Source: three-view drawing plus pictorial views. Frame: mm from the lowest corner of the part. A direction names the side the tool comes from. Give positions to 0.01 mm unless a question says otherwise; leave off trailing zeros. Loops run counter-clockwise (first coordinate to the right, second up) from the corner with the lowest first, then second, coordinate; pieces in that order, holes last. Notation, with made-up numbers: (24, 62.25) -> (46, 62.25) arc R6 cw to (46, 69.25) -> close; hole circle Ø8 at (34.5, 58). An arc over 180 degrees is marked (long way). One line per item, written item: value. Start each with the question number.
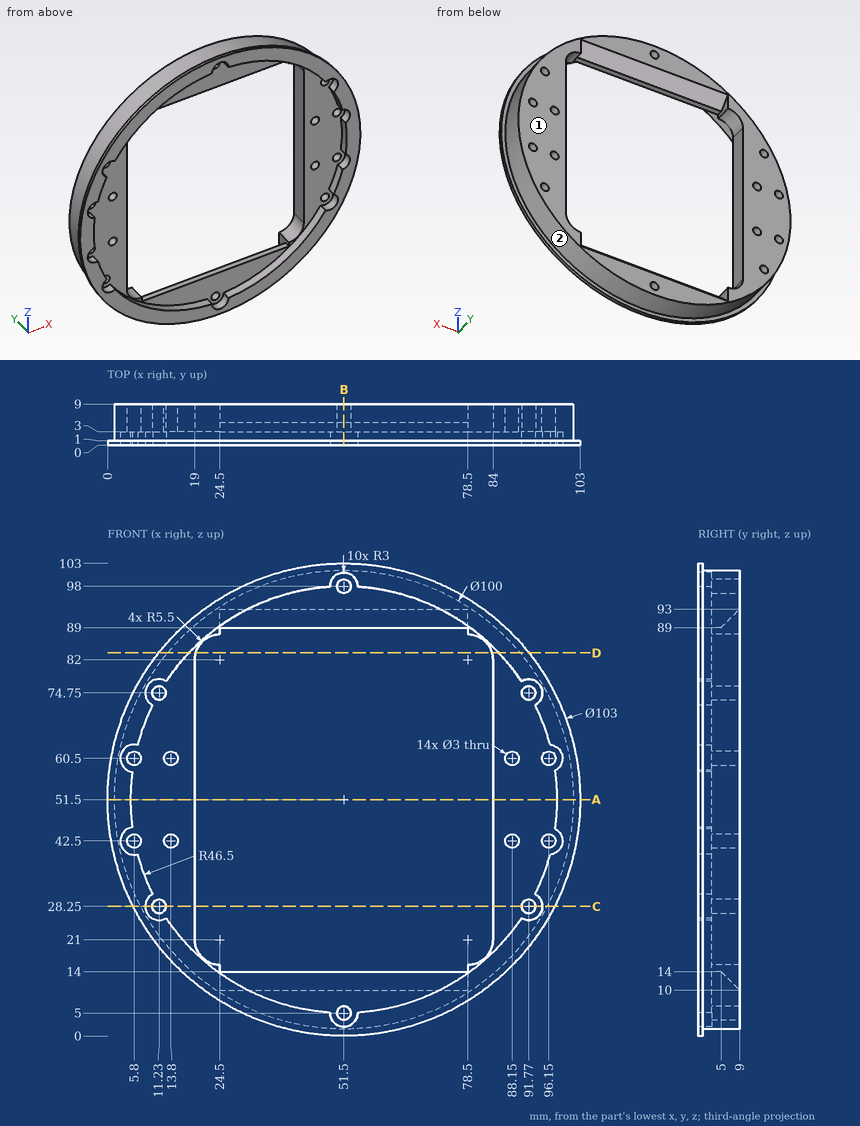
Item 1: Section A-A, the plane z = 51.5. Output: boundary loops of the cut face in (x, y).
Item 2: Section D-D, the plane z = 83.5. Output: boundary loops of the cut face in (x, y), then the cut area to 4 significant figures.
Item 3: Section C-C, the plane z = 28.25. Output: boundary loops of the cut face in (x, y).
Item 4: Pin query (flat end, axial travel): pin 1 (4 mm diameter, centred on x = 51.5, z = 5, fed in from -Y); pin 2 (1.6 mm diameter, centred on x = 44, y = 4, fed in from -Z); pin 3 (4.5 mm diameter, centred on y = 7, z = 13, fed in from -X); pin 4 (12 mm diameter, centred on x = 36.5, z = 81, fed in from -Y). Return the tip coordinate at first contact, or that it passes through.
Item 5: Ray query, line 1 along Z through (x, y) = (96.15, 7.65); line 2 along X through (y, z) = (4.5, 37.5); line 3 along Z through (x, y) = (5.8, 6.8) (1 decimal). Return the intervals inside material, ascending. Write a range as [from, to].
Item 6: Access query for the marked faces 1 and 2. Directions: +Z, -Z, +X, -X, +Y, -Y. A direction counts if a zero-diameter tool reaches every point of the face in a straight line with its end or side. Return the directions, or none.
Item 7: Section B-B, the plane x = 51.5. Output: boundary loops of the cut face in (y, z), then the cut area to 3 significant figures.
Geometry check:
1. outline: (0, 0) -> (5, 0) -> (5, 3) -> (19, 3) -> (19, 9) -> (1.5, 9) -> (1.5, 1) -> (0, 1) -> close; (84, 3) -> (98, 3) -> (98, 0) -> (103, 0) -> (103, 1) -> (101.5, 1) -> (101.5, 9) -> (84, 9) -> close
2. outline: (11.15, 0) -> (17.76, 0) -> (17.76, 3) -> (19.21, 3) -> (19.21, 9) -> (13.08, 9) -> (13.08, 1) -> (11.15, 1) -> close; (83.79, 3) -> (85.24, 3) -> (85.24, 0) -> (91.85, 0) -> (91.85, 1) -> (89.92, 1) -> (89.92, 9) -> (83.79, 9) -> close
2. area: 105.5 mm2
3. outline: (5.55, 0) -> (8.23, 0) -> (8.23, 3) -> (9.73, 3) -> (9.73, 9) -> (7.23, 9) -> (7.23, 1) -> (5.55, 1) -> close; (12.73, 3) -> (19, 3) -> (19, 9) -> (12.73, 9) -> close; (84, 3) -> (90.27, 3) -> (90.27, 9) -> (84, 9) -> close; (93.27, 3) -> (94.77, 3) -> (94.77, 0) -> (97.45, 0) -> (97.45, 1) -> (95.77, 1) -> (95.77, 9) -> (93.27, 9) -> close
4. pin 1: stops at y = 3
4. pin 2: stops at z = 1.95
4. pin 3: stops at x = 17.06
4. pin 4: passes through
5. line 1: z = [29, 41], [44, 59], [62, 74]
5. line 2: x = [3.5, 19], [84, 99.5]
5. line 3: z = [31.2, 41], [44, 59], [62, 71.8]
6. face 1: +Z, -Z, +X, -X, +Y
6. face 2: +Y
7. outline: (0, 0) -> (1, 0) -> (1, 1.5) -> (9, 1.5) -> (9, 3.5) -> (3, 3.5) -> (3, 2) -> (0, 2) -> close; (0, 101) -> (3, 101) -> (3, 99.5) -> (9, 99.5) -> (9, 101.5) -> (1, 101.5) -> (1, 103) -> (0, 103) -> close; (3, 6.5) -> (9, 6.5) -> (9, 10) -> (5, 14) -> (3, 14) -> close; (3, 89) -> (5, 89) -> (9, 93) -> (9, 96.5) -> (3, 96.5) -> close
7. area: 104 mm2
